```python
from build123d import *

# Parameters (mm, degrees)
PAD008_DEPTH    = 2.8
FILLET001_R     = 0.4
POCKET004_DEPTH = 2.801


with BuildPart() as part:
    # Sketch008 (on Face4 of ShapeBinder007) → Pad008 (new body)
    with BuildSketch(Plane(origin=(0, 20.211282, 0), x_dir=(-1, 0, 0), z_dir=(0, 1, 0))):
        with BuildLine():
            Line((37.8, 63.127675), (37.8, 60.327675))
            Line((37.8, 60.327675), (23.8, 60.327675))
            ThreePointArc((23.8, 60.327675), (23.4, 59.927675), (23.8, 59.527675))
            Line((23.8, 59.527675), (37.8, 59.527675))
            Line((37.8, 59.527675), (37.8, -33.872325))
            Line((37.8, -33.872325), (23.8, -33.872325))
            ThreePointArc((23.8, -33.872325), (23.4, -34.272325), (23.8, -34.672325))
            Line((23.8, -34.672325), (37.8, -34.672325))
            Line((37.8, -34.672325), (37.8, -37.472325))
            Line((37.8, -37.472325), (35.8, -38.222325))
            Line((35.8, -38.222325), (35.8, -37.472325))
            Line((35.8, -37.472325), (33, -37.472325))
            Line((33, -39.472325), (33, -37.472325))
            Line((25.535898, -37.472325), (33, -39.472325))
            Line((-25.535898, -37.472325), (25.535898, -37.472325))
            Line((-33, -39.472325), (-25.535898, -37.472325))
            Line((-33, -37.472325), (-33, -39.472325))
            Line((-35.8, -37.472325), (-33, -37.472325))
            Line((-35.8, -38.222325), (-35.8, -37.472325))
            Line((-37.8, -37.472325), (-35.8, -38.222325))
            Line((-37.8, -37.472325), (-37.8, -34.672325))
            Line((-37.8, -34.672325), (-23.8, -34.672325))
            ThreePointArc((-23.8, -34.672325), (-23.4, -34.272325), (-23.8, -33.872325))
            Line((-23.8, -33.872325), (-37.8, -33.872325))
            Line((-37.8, -33.872325), (-37.8, 59.527675))
            Line((-23.8, 59.527675), (-37.8, 59.527675))
            ThreePointArc((-23.8, 59.527675), (-23.4, 59.927675), (-23.8, 60.327675))
            Line((-37.8, 60.327675), (-23.8, 60.327675))
            Line((-37.8, 60.327675), (-37.8, 63.127675))
            Line((-37.8, 63.127675), (-35.8, 63.877675))
            Line((-35.8, 63.877675), (-35.8, 63.127675))
            Line((-35.8, 63.127675), (-33, 63.127675))
            Line((-33, 65.127675), (-33, 63.127675))
            Line((-25.535898, 63.127675), (-33, 65.127675))
            Line((25.535898, 63.127675), (-25.535898, 63.127675))
            Line((33, 65.127675), (25.535898, 63.127675))
            Line((33, 63.127675), (33, 65.127675))
            Line((35.8, 63.127675), (33, 63.127675))
            Line((35.8, 63.877675), (35.8, 63.127675))
            Line((37.8, 63.127675), (35.8, 63.877675))
        make_face()
    extrude(amount=-PAD008_DEPTH)

    # Fillet001
    fillet001_edges = [part.edges().sort_by_distance(p)[0] for p in [
        (-33, 18.811282, 65.127675),
        (-37.8, 18.811282, 63.127675),
        (-37.8, 18.811282, 60.327675),
        (-37.8, 18.811282, 59.527675),
        (-37.8, 18.811282, -33.872325),
        (-37.8, 18.811282, -34.672325),
        (-37.8, 18.811282, -37.472325),
        (-33, 18.811282, -39.472325),
        (33, 18.811282, -39.472325),
        (37.8, 18.811282, -37.472325),
        (37.8, 18.811282, -34.672325),
        (37.8, 18.811282, -33.872325),
        (33, 18.811282, 65.127675),
        (37.8, 18.811282, 63.127675),
        (37.8, 18.811282, 60.327675),
        (37.8, 18.811282, 59.527675),
    ]]
    fillet(fillet001_edges, radius=FILLET001_R)

    # Sketch017 (on Face2 of Fillet001) → Pocket004 (cut, through all)
    with BuildSketch(Plane(origin=(0, 20.211282, 0), x_dir=(-1, 0, 0), z_dir=(0, 1, 0))):
        with BuildLine():
            ThreePointArc((-11.75, 60.327675), (-12.81066, 59.888335), (-13.25, 58.827675))
            ThreePointArc((-13.25, 58.827675), (-13.24452, 58.699573), (-13.22812, 58.572408))
            ThreePointArc((-13.22812, 45.082943), (-12.65, 51.827675), (-13.22812, 58.572408))
            ThreePointArc((-13.22812, 45.082943), (-13.24452, 44.955777), (-13.25, 44.827675))
            ThreePointArc((-13.25, 44.827675), (-12.81066, 43.767015), (-11.75, 43.327675))
            Line((11.75, 43.327675), (-11.75, 43.327675))
            ThreePointArc((11.75, 43.327675), (12.81066, 43.767015), (13.25, 44.827675))
            ThreePointArc((13.25, 44.827675), (13.24452, 44.955777), (13.22812, 45.082943))
            ThreePointArc((13.22812, 58.572408), (12.65, 51.827675), (13.22812, 45.082943))
            ThreePointArc((13.22812, 58.572408), (13.24452, 58.699573), (13.25, 58.827675))
            ThreePointArc((13.25, 58.827675), (12.81066, 59.888335), (11.75, 60.327675))
            Line((-11.75, 60.327675), (11.75, 60.327675))
        make_face()
        with BuildLine():
            ThreePointArc((-14.7587, 44.73481), (-14.09424, 51.827675), (-14.7587, 58.92054))
            ThreePointArc((-14.7587, 58.92054), (-15.342865, 59.318975), (-15.7413, 58.73481))
            ThreePointArc((-15.7413, 44.92054), (-15.09424, 51.827675), (-15.7413, 58.73481))
            ThreePointArc((-15.7413, 44.92054), (-15.342865, 44.336375), (-14.7587, 44.73481))
        make_face()
        with BuildLine():
            ThreePointArc((14.7587, 58.92054), (14.09424, 51.827675), (14.7587, 44.73481))
            ThreePointArc((14.7587, 44.73481), (15.342865, 44.336375), (15.7413, 44.92054))
            ThreePointArc((15.7413, 58.73481), (15.09424, 51.827675), (15.7413, 44.92054))
            ThreePointArc((15.7413, 58.73481), (15.342865, 59.318975), (14.7587, 58.92054))
        make_face()
    extrude(amount=-POCKET004_DEPTH, mode=Mode.SUBTRACT)


solid = part.part
```
Here's how the part is built. I have some questions about the finished solid (model axes, mm). A direction names the side the tool comes from. Coordinates: 2 decimals unless noted, no trailing zeros. Loops run counter-clockwise (first coordinate to the right, second up) from the corner with the lowest first, then second, coordinate; pieces in that order, holes last. Notation, with made-up numbers: (80.5, 66) - (107.5, 66) arc R33 ccw to (107.5, 97) - close; hole circle Ø8 at (36, 78). An arc over 180 degrees is marked (long way). Answer as CSV lines item,"result".
Q1. If I drill on L1, parallel to Z at x = -24, y = 19.55; L2, parallel to X at y = 18.9, z = 46.5; L3, parallel to Z at x = 31, y = 19.75, over which ranges is the centre line in solid material (lowest first)? Write a range as [from, to].
Response:
L1,"[-37.47, -34.67], [-33.87, 59.53], [60.33, 63.13]"
L2,"[-37.8, -15.48], [-14.47, -13.01], [13.01, 14.47], [15.48, 37.8]"
L3,"[-38.94, -34.67], [-33.87, 59.53], [60.33, 64.59]"
Q2. For pin 1 (1.4 mm diameter, centred on x = -35, y = 18.5, fed in from +Z); pin 2 (1.4 mm diameter, centred on x = 28.5, y = 18.5, fed in from -Z); pin 3 (1.2 mm diameter, centred on y = 19.5, z = 63.5, fed in from +X), each with a flat end and sliding along its axis, tell me the tip position at first contact or that it passes through.
Response:
pin 1,"z = 63.13"
pin 2,"z = -38.45"
pin 3,"x = 37.8"
Q3. We'd pull the mould along X, two halves only. Please class faces 1 (the face through (37.8, 19, 62)), 2 (the face through (-12.65, 18.83, 51.92)), 3 (the face through (31, 19, -34.672)): pulls with the +X half, pulls with the -X half, needs draft (parallel to the pull), parting line crosses it, or undercut.
Response:
face 1,"pulls with the +X half"
face 2,"undercut"
face 3,"needs draft"
Q4. For faces 4 (the face through (-14.094, 18.831, 51.928)), 5 (the face through (-34, 19, -37.472)), 6 (the face through (-29.06, 18.83, 64.07)), which set-ups out of +Z, -Z, +X, -X, +Y, -Y let a thin tool reach every point of the face, with its end or its side?
Response:
face 4,"+Y, -Y"
face 5,"-Z, +Y, -Y"
face 6,"+Z, +Y, -Y"
Q5. If we section it at B-B, the plane y = 18: Give the number of separate pieces and of enclosed holes in the cut face, and give its area (3 significant figures).
Response:
separate pieces,"1"
enclosed holes,"3"
area,"7,120 mm2"
Q6. If we section it at C-C, the plane x = 20: Write out the boundary of the cut face in (y, z).
Response:
outline,"(17.41, -37.47) - (20.21, -37.47) - (20.21, 63.13) - (17.41, 63.13) - close"
Q7. If we section it at A-A, the plane x = -6: Write out the boundary of the cut face in (y, z), and give its area (3 significant figures).
Response:
outline,"(17.41, -37.47) - (20.21, -37.47) - (20.21, 43.33) - (17.41, 43.33) - close; (17.41, 60.33) - (20.21, 60.33) - (20.21, 63.13) - (17.41, 63.13) - close"
area,"234 mm2"
